Geometry check sheet. Reference: drawing and pictorial views, mm from the part's lowest x, y, z. A direction names the side the tool comes from. Round coordinates to 2 decimals unless told otherwise and drop trailing zeros. Loops run counter-clockwise (first coordinate to the right, second up) from the corner with the lowest first, then second, coordinate; pieces in that order, holes last. Notation, with made-up numbers: (-10, 19) - (43, 19) arc R36 ccw to (43, 58) - close; hole circle Ø9 at (4, 89). An arc over 180 degrees is marked (long way). Put each result on its own line as item: value. Start each with the question number.
Item 1: Section check A-A, the plane z = 10. Record the cut outline in (x, y) (1 decimal).
Item 2: Draft check along Y on the marked faces 1, 2 and 3. Enter one of: pulls with the +Y half, pulls with the -Y half, needs draft (parallel to the pull), parting line crosses it, or undercut.
Item 3: Material ranges on line 1 along Y through (x, z) = (3.5, 2.25); line 2 along X through (y, z) = (8.25, 16.75); line 3 along Y through (x, z) = (6.5, 8.5), recorded low to high.
Item 4: Section check C-C, the plane x = 17. Record the cut outline in (y, z) (1 decimal), and give its area (3 significant figures).
Item 5: Section check D-D, the plane z = 4. Record the cut outline in (x, y).
Item 6: Section check B-B, the plane y = 12. Record the cut outline in (x, z).
Item 7: Tool access check on the marked faces 4, 5 and 6. Record the directions out of +Z, -Z, +X, -X, +Y, -Y that give a thin tool (end or side, any length) a straight path to the whole face; none if there is none.
Item 8: Gauge pin test, flat ends, axial feed: pin 1 Ø6 at (y, z) = (11.62, 10) entering from -X; pin 2 Ø1 at (x, z) = (13, 7) entering from +Y; pin 3 Ø10 at (x, y) = (13, 6.5) entering from +Z; pin 4 Ø2.5 at (x, z) = (8.09, 10) entering from +Y. Record the tip position at first contact, or that the pin passes through.
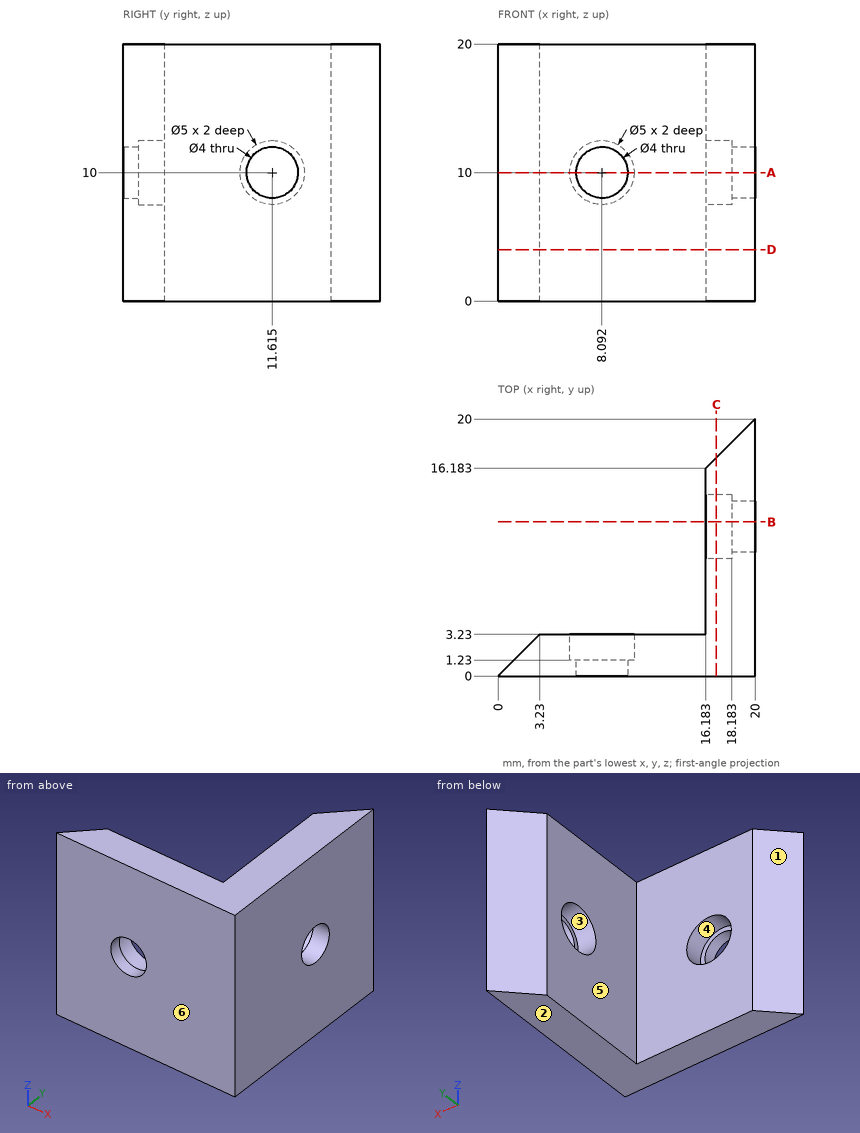
Check result:
1. outline: (0, 0) - (6.1, 0) - (6.1, 1.2) - (5.6, 1.2) - (5.6, 3.2) - (3.2, 3.2) - close; (10.1, 0) - (20, 0) - (20, 9.6) - (18.2, 9.6) - (18.2, 9.1) - (16.2, 9.1) - (16.2, 3.2) - (10.6, 3.2) - (10.6, 1.2) - (10.1, 1.2) - close; (16.2, 14.1) - (18.2, 14.1) - (18.2, 13.6) - (20, 13.6) - (20, 20) - (16.2, 16.2) - close
2. face 1: pulls with the +Y half
2. face 2: needs draft
2. face 3: undercut
3. line 1: 0 to 3.23
3. line 2: 16.18 to 20
3. line 3: 0 to 1.23
4. outline: (0, 0) - (17, 0) - (17, 20) - (0, 20) - close; hole circle Ø5 at (11.6, 10)
4. area: 320 mm²
5. outline: (0, 0) - (20, 0) - (20, 20) - (16.18, 16.18) - (16.18, 3.23) - (3.23, 3.23) - close
6. outline: (16.18, 0) - (20, 0) - (20, 8.04) - (18.18, 8.04) - (18.18, 7.53) - (16.18, 7.53) - close; (16.18, 12.47) - (18.18, 12.47) - (18.18, 11.96) - (20, 11.96) - (20, 20) - (16.18, 20) - close
7. face 4: +Y
7. face 5: +Z, -Z, -X, +Y
7. face 6: +Z, -Z, +X, -X, -Y
8. pin 1: x = 16.18
8. pin 2: y = 3.23
8. pin 3: z = 20
8. pin 4: through
